```python
from build123d import *

# Parameters (mm, degrees)
F0_R     = 11.6
F0_W     = 2.1
F0_H     = 0.3
F0_R_2   = 2.1
F1_DEPTH = 1


with BuildPart() as f1:
    # F0 (on Front) → F1 (new body)
    with BuildSketch(Plane.XZ):
        Circle(F0_R)
        with Locations((-9.05, 0)):
            Rectangle(F0_W, F0_H, mode=Mode.SUBTRACT)
        Circle(F0_R_2, mode=Mode.SUBTRACT)
        with Locations((9.05, 0)):
            Rectangle(F0_W, F0_H, mode=Mode.SUBTRACT)
    extrude(amount=F1_DEPTH)


solid = f1.part
```
Verification items for the finished model (mm, model axes). A direction names the side the tool comes from. Coordinates: 2 decimals unless noted, no trailing zeros. Write each loop counter-clockwise with the first axis right and the second up, starting at its lowest first coordinate (ties: lowest second). Pieces come first, ordered by that corner, then holes. Notation, with made-up numbers: M 24,-31.5 L 46,-31.5 A28 cw 46,-1.5 Z; hole C 58.25,48 d3. An arc over 180 degrees is marked long. Answer as a JSON object with one key per item and string values. Group by question number.
(1) Gauge pin test, flat ends, axial feed: pin 1 (6 mm diameter, centred on x = 2, z = -1.5, fed in from +Y); pin 2 (0.5 mm diameter, centred on x = -9, y = -0.5, fed in from -Z). Record the tip position at first contact, or that the pin passes through.
(2) Material ranges on line 1 (Z direction, x = 0, y = -0.7); line 2 (Z direction, x = -9, y = -0.6); line 3 (X direction, y = -0.1, z = -6.25), recorded low to high.
(3) Cross-section at C-C, the plane y = -0.2. Record the cut outline in (x, z).
(4) Cross-section at A-A, the plane x = 0. Record the cut outline in (y, z).
(5) Tool access check on faces 4 (the face through (-9.1, -0.5, -0.15)), 5 (the face through (2.4, -1, 0.2)). Record the directions out of +Z, -Z, +X, -X, +Y, -Y that give a thin tool (end or side, any length) a straight path to the whole face; none if there is none.
(6) Release check for a two-part mould opening along Z. For faces 1 (the face through (2.4, 0, 0.2)), 2 (the face through (9, -0.5, -0.15)), 3 (the face through (-11.59, -0.49, 0.51)) record: +Z half, -Z half, draft (parallel to the pull), parting line (faces both ways), or undercut.
(7) Cross-section at B-B, the plane z = -1.75. Record the cut outline in (x, y).
(8) Cross-section at D-D, the plane z = -8. Record the cut outline in (x, y), and give its area (3 significant figures).
Reply:
{
 "1": {"pin 1": "y = 0", "pin 2": "z = -7.62"},
 "2": {"line 1": "-11.6 to -2.1, 2.1 to 11.6", "line 2": "-7.32 to -0.15, 0.15 to 7.32", "line 3": "-9.77 to 9.77"},
 "3": {"outline": "C 0,0 d23.2; hole M -10.1,-0.15 L -8,-0.15 L -8,0.15 L -10.1,0.15 Z; hole C 0,0 d4.2; hole M 8,-0.15 L 10.1,-0.15 L 10.1,0.15 L 8,0.15 Z"},
 "4": {"outline": "M -1,-11.6 L 0,-11.6 L 0,-2.1 L -1,-2.1 Z; M -1,2.1 L 0,2.1 L 0,11.6 L -1,11.6 Z"},
 "5": {"face 4": "+Y, -Y", "face 5": "+Z, -Z, +X, -X, -Y"},
 "6": {"face 1": "draft", "face 2": "undercut", "face 3": "parting line"},
 "7": {"outline": "M -11.47,-1 L -1.16,-1 L -1.16,0 L -11.47,0 Z; M 1.16,-1 L 11.47,-1 L 11.47,0 L 1.16,0 Z"},
 "8": {"outline": "M -8.4,-1 L 8.4,-1 L 8.4,0 L -8.4,0 Z", "area": "16.8 mm²"}
}
